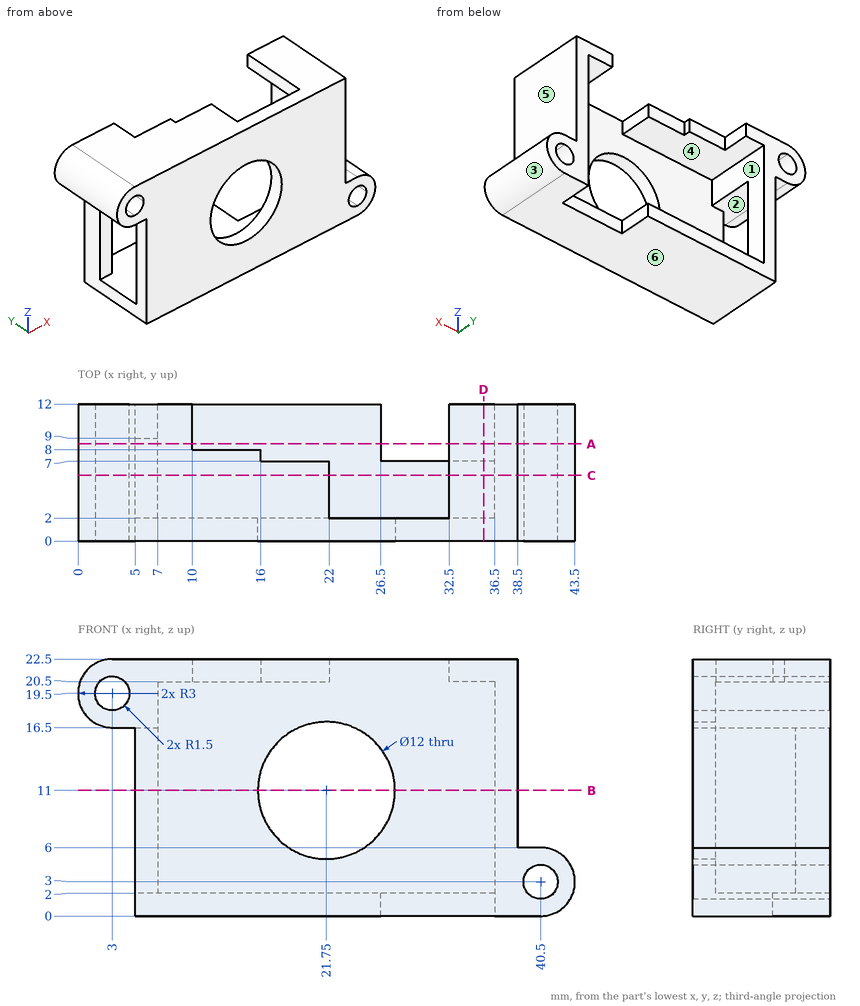
Check sheet for the drawn part. Datum: minimum x, y, z corner. Units: mm. A direction names the side the tool comes from. Round coordinates to 2 decimals unless told otherwise and drop trailing zeros. Loops run counter-clockwise (first coordinate to the right, second up) from the corner with the lowest first, then second, coordinate; pieces in that order, holes last. Notation, with made-up numbers: M 44.5,46.25 L 76.5,46.25 A26 cw 76.5,84.25 Z; hole C 81,63 d8. An arc over 180 degrees is marked long. One line per question, with ' | ' between items. Start each with the question number.
Item 1: Section check A-A (y = 8.5). Record the boundary of the cut face in (x, z).
Item 2: Set-up check for the marked faces 1, 2 and 3: record each of +Z, -Z, +X, -X, +Y, -Y from which the full face is reachable in a straight line by a thin tool's end or side.
Item 3: Release check for a two-part mould opening along X. For the marked faces 4, 5 and 6 record: released by +X, released by -X, zero draft, split by the parting line, or undercut.
Item 4: Section check B-B (z = 11). Record the boundary of the cut face in (x, y).
Item 5: Scan lines: probe 1 along X at (y, z) = (10, 19.5); probe 2 along Z at (x, y) = (6.5, 3); probe 3 along Z at (x, y) = (21.75, 1.4). Record each from-to range of solid material in increasing order.
Item 6: Section check D-D (x = 35.5). Record the boundary of the cut face in (y, z), and give its area (3 significant figures).
Item 7: Section check C-C (y = 5.75). Record the boundary of the cut face in (x, z).
Item 8: Gauge pin test, flat ends, axial feed: pin 1 Ø1 at (x, z) = (18, 22) entering from +Y; pin 2 Ø0.6 at (x, z) = (14, 21.5) entering from +Y; pin 3 Ø3 at (x, y) = (28, 4) entering from +Z. Record the tip position at first contact, or that the pin passes through.
Worked out:
1) outline: M 3,16.5 L 7,16.5 L 7,20.5 L 10,20.5 L 10,22.5 L 3,22.5 A3 ccw Z; M 5,0 L 26.5,0 L 26.5,2 L 5,2 Z; M 32.5,20.5 L 36.5,20.5 L 36.5,0 L 40.5,0 A3 ccw 40.5,6 L 38.5,6 L 38.5,22.5 L 32.5,22.5 Z; hole M 3,18 A1.5 ccw 4.5,19.5 A1.5 ccw long Z; hole M 40.5,1.5 A1.5 ccw 42,3 A1.5 ccw long Z
2) face 1: +Y | face 2: -X | face 3: +X, +Y, -Y
3) face 4: undercut | face 5: released by +X | face 6: zero draft
4) outline: M 5,0 L 15.75,0 L 15.75,2 L 5,2 Z; M 5,9 L 7,9 L 7,12 L 5,12 Z; M 27.75,0 L 38.5,0 L 38.5,12 L 36.5,12 L 36.5,2 L 27.75,2 Z
5) probe 1: 0 to 1.5, 4.5 to 7, 36.5 to 38.5 | probe 2: 0 to 2, 16.5 to 22.5 | probe 3: 0 to 5, 17 to 22.5
6) outline: M 0,0 L 7,0 L 7,2 L 2,2 L 2,20.5 L 12,20.5 L 12,22.5 L 0,22.5 Z | area: 75.0 mm^2
7) outline: M 3,16.5 L 7,16.5 L 7,20.5 L 22,20.5 L 22,22.5 L 3,22.5 A3 ccw Z; M 5,0 L 40.5,0 A3 ccw 40.5,6 L 38.5,6 L 38.5,22.5 L 32.5,22.5 L 32.5,20.5 L 36.5,20.5 L 36.5,2 L 5,2 Z; hole M 3,18 A1.5 ccw 4.5,19.5 A1.5 ccw long Z; hole M 40.5,1.5 A1.5 ccw 42,3 A1.5 ccw long Z
8) pin 1: y = 7 | pin 2: y = 8 | pin 3: z = 2
